For this review, use the dimensioned drawing (mm, ordinates from the lowest corner) and the shaded views. Round coordinates to 2 decimals unless told otherwise and drop trailing zeros. Order: outer loops, then holes, each group sorted by start corner. A loop starts at its lowest first (then second) coordinate and runs counter-clockwise, first axis right, second up. Notation, with made-up numbers: (56.25, 12.25) -> (63.25, 12.25) arc R34 ccw to (63.25, 48.25) -> close; hole circle Ø7 at (89.5, 9.5). An arc over 180 degrees is marked (long way). Use a Markdown table: item, result. Add a question column.
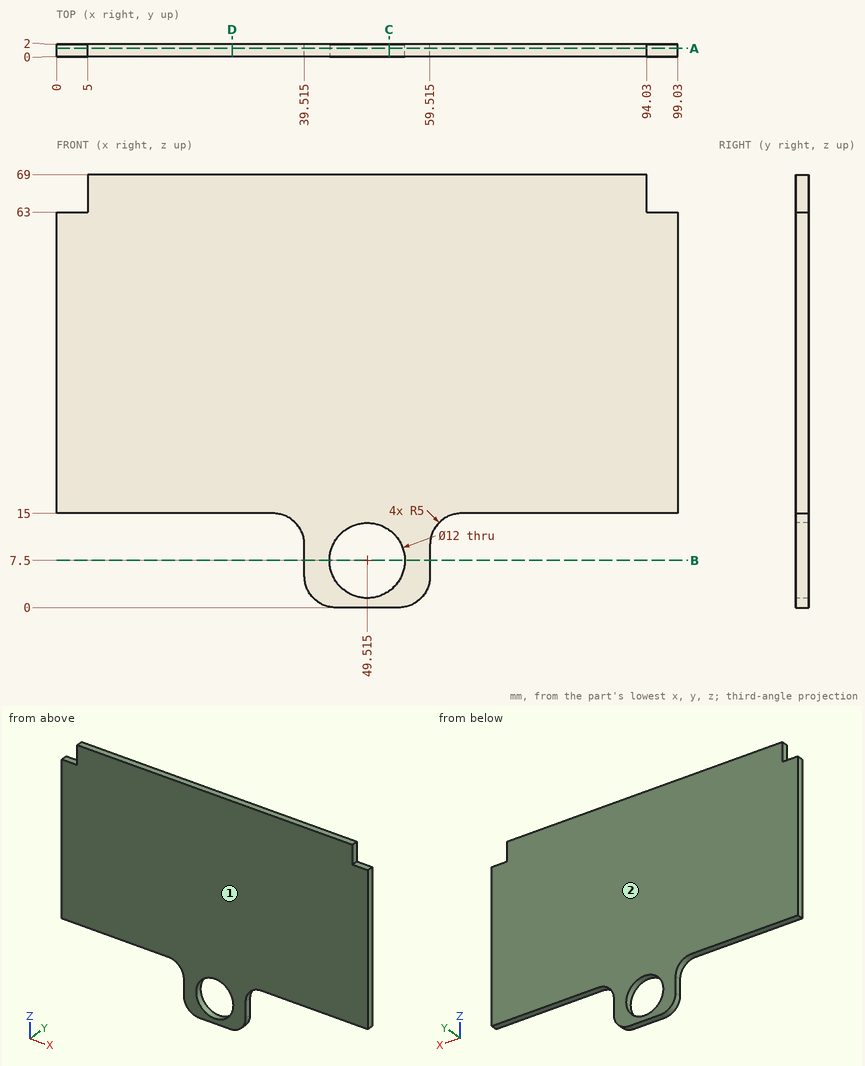
Q1. Add section D-D (x = 28). Write out the cut boundary in (y, z).
Q2. Wall thickness on line 1 (X direction, y = 0.7, z = 7.5) (1 decimal); line 2 (Z direction, x = 49, y = 1.4); line 3 (Z direction, x = 25.5, y = 1.35): over which ranges is each line inside the solid? List them lowest first. Write a range as [from, to].
Q3. Insertion check: pin 1 (0.6 mm diameter, centred on y = 0.5, z = 67, fed in from -X); pin 2 (1 mm diameter, centred on x = 58, y = 1, fed in from -Z); pin 3 (1 mm diameter, centred on x = 95.5, y = 1, fed in from +Z). Each pin has a flat end and moves straight along its axis. Give the tip position at first contact, or say it passes through.
Q4. Add section C-C (x = 53). Write out the cut boundary in (y, z) (1 decimal).
Q5. Mouldability with a two-part tool opening along Y and no side actions: class the marked faces 1 and 2 as pulls with the +Y half, pulls with the -Y half, needs draft (parallel to the pull), parting line crosses it, or undercut.
Q6. Add section A-A (y = 1.3). Write out the cut boundary in (x, z) (1 decimal).
Q7. Add section B-B (z = 7.5). Write out the cut boundary in (x, y) (1 decimal).
Report:
| question | item | result |
|---|---|---|
| 1 | outline | (0, 15) -> (2, 15) -> (2, 69) -> (0, 69) -> close |
| 2 | line 1 | x = [39.5, 43.5], [55.5, 59.5] |
| 2 | line 2 | z = [0, 1.52], [13.48, 69] |
| 2 | line 3 | z = [15, 69] |
| 3 | pin 1 | stops at x = 5 |
| 3 | pin 2 | stops at z = 0.99 |
| 3 | pin 3 | stops at z = 63 |
| 4 | outline | (0, 0) -> (2, 0) -> (2, 2.6) -> (0, 2.6) -> close; (0, 12.4) -> (2, 12.4) -> (2, 69) -> (0, 69) -> close |
| 5 | face 1 | pulls with the -Y half |
| 5 | face 2 | pulls with the +Y half |
| 6 | outline | (0, 15) -> (34.5, 15) arc R5 cw to (39.5, 10) -> (39.5, 5) arc R5 ccw to (44.5, 0) -> (54.5, 0) arc R5 ccw to (59.5, 5) -> (59.5, 10) arc R5 cw to (64.5, 15) -> (99, 15) -> (99, 63) -> (94, 63) -> (94, 69) -> (5, 69) -> (5, 63) -> (0, 63) -> close; hole circle Ø12 at (49.5, 7.5) |
| 7 | outline | (39.5, 0) -> (43.5, 0) -> (43.5, 2) -> (39.5, 2) -> close; (55.5, 0) -> (59.5, 0) -> (59.5, 2) -> (55.5, 2) -> close |
